Source: CAD feature listing. Evaluate the final solid. Frame: model axes, mm. Face numbers are marked on the shaded views. A direction names the side the tool comes from. Round coordinates to 2 decimals unless told otherwise and drop trailing zeros. Write each loop counter-clockwise with the first axis right and the second up, starting at its lowest first coordinate (ties: lowest second). Pieces come first, ordered by that corner, then holes. Notation, with made-up numbers: M 30,-17.75 L 59,-17.75 A22 ccw 59,9.25 Z; hole C -25,73.5 d11. An arc over 180 degrees is marked long. Answer in a Markdown table with one row per item.
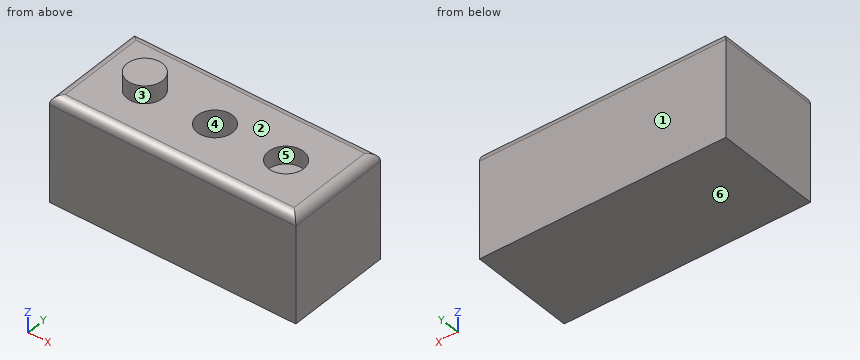
from build123d import *

# Parameters (mm, degrees)
F0_W     = 140
F0_H     = 60
F1_DEPTH = 60
F3_R     = 10
F6_DEPTH = 10
F4_R     = 10
F7_DEPTH = 25
F5_R     = 10
F8_DEPTH = 10
F9_R     = 5


with BuildPart() as f1:
    # F0 (on Top) → F1 (new body)
    with BuildSketch(Plane.XY):
        Rectangle(F0_W, F0_H)
    extrude(amount=F1_DEPTH)

    # F3 (on face) → F6 (join)
    with BuildSketch(Plane.XY.offset(60)):
        with Locations((-39.604324, -0.323002)):
            Circle(F3_R)
    extrude(amount=F6_DEPTH)

    # F4 (on face) → F7 (cut)
    with BuildSketch(Plane.XY.offset(60)):
        Circle(F4_R)
    extrude(amount=-F7_DEPTH, mode=Mode.SUBTRACT)

    # F5 (on face) → F8 (cut)
    with BuildSketch(Plane.XY.offset(60)):
        with Locations((40.830696, -0.571058)):
            Circle(F5_R)
    extrude(amount=-F8_DEPTH, mode=Mode.SUBTRACT)

    # F9
    f9_edges = [f1.edges().sort_by_distance(p)[0] for p in [
        (-70, 0, 60),
        (70, 0, 60),
        (0, -30, 60),
        (0, 30, 60),
    ]]
    fillet(f9_edges, radius=F9_R)


solid = f1.part
Q1. Contact query for flat-ended pins moving along their axis: pin 1 Ø6 at (x, y) = (11.5, 18.5) entering from +Z; pin 2 Ø10 at (y, z) = (-15.5, 58) entering from +X. Output: stop coordinate, or through.
Solutions:
| item | result |
|---|---|
| pin 1 | stops at z = 60 |
| pin 2 | stops at x = 70 |
Q2. Pull-direction query (Y, two-part tool) for the marked faces 1, 2, 3 and 4; classes: pulls with the +Y half, pulls with the -Y half, needs draft (parallel to the pull), parting line crosses it, or undercut.
Solutions:
| item | result |
|---|---|
| face 1 | pulls with the +Y half |
| face 2 | needs draft |
| face 3 | parting line crosses it |
| face 4 | undercut |
Q3. Section B-B (y = -17). Return loops of the section in (x, z), and give its area (3 significant figures).
Solutions:
| item | result |
|---|---|
| outline | M -70,0 L 70,0 L 70,55 A5 ccw 65,60 L -65,60 A5 ccw -70,55 Z |
| area | 8,390 mm2 |
Q4. Section A-A (x = 0). Return loops of the section in (y, z), and give its area (3 significant figures).
Solutions:
| item | result |
|---|---|
| outline | M -30,0 L 30,0 L 30,55 A5 ccw 25,60 L 10,60 L 10,35 L -10,35 L -10,60 L -25,60 A5 ccw -30,55 Z |
| area | 3,090 mm2 |
Q5. Section C-C (z = 36.5). Return loops of the section in (x, y).
Solutions:
| item | result |
|---|---|
| outline | M -70,-30 L 70,-30 L 70,30 L -70,30 Z; hole C 0,0 d20 |
Q6. Section D-D (z = 52.5). Return loops of the section in (x, y).
Solutions:
| item | result |
|---|---|
| outline | M -70,-30 L 70,-30 L 70,30 L -70,30 Z; hole C 0,0 d20; hole C 40.83,-0.57 d20 |
Q7. Material intervals for probe 1 along Y at (x, z) = (0, 54); probe 2 along Z at (x, y) = (-44.5, -14); probe 3 along Y at (x, z) = (8, 45.5), sorted ascending.
Solutions:
| item | result |
|---|---|
| probe 1 | y = -30 to -10, 10 to 30 |
| probe 2 | z = 0 to 60 |
| probe 3 | y = -30 to -6, 6 to 30 |
Q8. Access query for the marked faces 5 and 6. Directions: +Z, -Z, +X, -X, +Y, -Y. A direction counts if a zero-diameter tool reaches every point of the face in a straight line with its end or side. Return the directions, or none.
Solutions:
| item | result |
|---|---|
| face 5 | +Z |
| face 6 | -Z, +X, -X, +Y, -Y |
